Check sheet for the modelled part. Datum: model origin and axes. Units: mm. A direction names the side the tool comes from. Give positions to 0.01 mm unless a question says otherwise; leave off trailing zeros. Order: outer loops, then holes, each group sorted by start corner. A loop starts at its lowest first (then second) coordinate and runs counter-clockwise, first axis right, second up. Notation, with made-up numbers: (-15, 83.25) -> (29, 83.25) arc R35 cw to (29, 121.25) -> close; hole circle Ø2 at (84, 7.25). An arc over 180 degrees is marked (long way). Answer in a Markdown table with one row per item. Add a question column.
(1) Release check for a two-part mould opening along Y. For faces 4 (the face through (106, 26, 37)), 5 (the face through (65, 44, 37)), 6 (the face through (27.3, 40.6, 36.9)) record: released by +Y, released by -Y, zero draft, split by the parting line, or undercut.
(2) Cross-section at A-A (y = 41.5). Record the cut outline in (x, z).
(3) Set-up check for faces 1 (the face through (102.15, 26, 41)), 2 (the face through (30.95, 26, 41)), 3 (the face through (66, 38.3, 41)): record each of +Z, -Z, +X, -X, +Y, -Y from which the full face is reachable in a straight line by a thin tool's end or side.
(4) Go/stop test with flat-tipped pins: pin 1 (1.1 mm diameter, centred on y = 28.5, z = 44.5, fed in from +X); pin 2 (3 mm diameter, centred on y = 25.5, z = 41, fed in from -X); pin 3 (5 mm diameter, centred on x = 68, z = 42, fed in from -Y). Record where each tip stops, or that it passes through.
(5) Cross-section at C-C (x = 71). Record the cut outline in (y, z).
(6) Cross-section at B-B (x = 103.6). Record the cut outline in (y, z), then the cut area to 3 significant figures.
(7) Cross-section at D-D (z = 39.75). Record the cut outline in (x, y).
(8) Thickness scan on L1, parallel to Y at x = 103.6, z = 37.1; L2, parallel to Y at x = 90, z = 44; L3, parallel to X at y = 19.5, z = 42.25. Record the ranges inside material, lowest first. Write a range as [from, to].
```python
from build123d import *

# Parameters (mm, degrees)
SKETCH031_W     = 80
SKETCH031_H     = 36
PAD009_DEPTH    = 1.7
SKETCH032_W     = 71.2
SKETCH032_H     = 25.2
PAD010_DEPTH    = 7
SKETCH033_R     = 1.5
POCKET008_DEPTH = 1.701
SKETCH034_W     = 66
SKETCH034_H     = 16
POCKET009_DEPTH = 1


with BuildPart() as part:
    # Sketch031 → Pad009 (new body)
    with BuildSketch(Plane.XY):
        with Locations((40, 18)):
            Rectangle(SKETCH031_W, SKETCH031_H)
    extrude(amount=PAD009_DEPTH)

    # Sketch032 (on Face6 of Pad009) → Pad010 (join)
    with BuildSketch(Plane.XY.offset(1.7)):
        with Locations((40.55, 17.7)):
            Rectangle(SKETCH032_W, SKETCH032_H)
    extrude(amount=PAD010_DEPTH)

    # Sketch033 (on Face5 of Pad010) → Pocket008 (cut, through all)
    with BuildSketch(Plane.XY.offset(1.7)):
        with Locations((2.5, 33.5)):
            Circle(SKETCH033_R)
        with Locations((2.5, 2.28424)):
            Circle(SKETCH033_R)
        with Locations((77.6, 33.5)):
            Circle(SKETCH033_R)
        with Locations((77.6, 2.28424)):
            Circle(SKETCH033_R)
    extrude(amount=-POCKET008_DEPTH, mode=Mode.SUBTRACT)

    # Sketch034 (on Face15 of Pocket008) → Pocket009 (cut)
    with BuildSketch(Plane.XY.offset(8.7)):
        with Locations((40.55, 17.7)):
            Rectangle(SKETCH034_W, SKETCH034_H)
    extrude(amount=-POCKET009_DEPTH, mode=Mode.SUBTRACT)


with BuildPart() as part_1:
    # Body009 placement: moved
    add(part.part.moved(Location((26, 8, 36))))


solid = part_1.part
```
Answer below:
| question | item | result |
|---|---|---|
| 1 | face 4 | zero draft |
| 1 | face 5 | released by +Y |
| 1 | face 6 | undercut |
| 2 | outline | (26, 36) -> (27, 36) -> (27, 37.7) -> (26, 37.7) -> close; (30, 36) -> (102.1, 36) -> (102.1, 37.7) -> (30, 37.7) -> close; (105.1, 36) -> (106, 36) -> (106, 37.7) -> (105.1, 37.7) -> close |
| 3 | face 1 | +Z, +X, +Y, -Y |
| 3 | face 2 | +Z, -X, +Y, -Y |
| 3 | face 3 | +Z, +X, -X, +Y |
| 4 | pin 1 | stops at x = 102.15 |
| 4 | pin 2 | stops at x = 30.95 |
| 4 | pin 3 | stops at y = 13.1 |
| 5 | outline | (8, 36) -> (44, 36) -> (44, 37.7) -> (38.3, 37.7) -> (38.3, 44.7) -> (33.7, 44.7) -> (33.7, 43.7) -> (17.7, 43.7) -> (17.7, 44.7) -> (13.1, 44.7) -> (13.1, 37.7) -> (8, 37.7) -> close |
| 6 | outline | (8, 36) -> (8.78, 36) -> (8.78, 37.7) -> (8, 37.7) -> close; (11.78, 36) -> (40, 36) -> (40, 37.7) -> (11.78, 37.7) -> close; (43, 36) -> (44, 36) -> (44, 37.7) -> (43, 37.7) -> close |
| 6 | area | 51.0 mm² |
| 7 | outline | (30.95, 13.1) -> (102.15, 13.1) -> (102.15, 38.3) -> (30.95, 38.3) -> close |
| 8 | L1 | y = [8, 8.78], [11.78, 40], [43, 44] |
| 8 | L2 | y = [13.1, 17.7], [33.7, 38.3] |
| 8 | L3 | x = [30.95, 102.15] |
